Check sheet for the drawn part. Datum: minimum x, y, z corner. Units: mm. A direction names the side the tool comes from. Give positions to 0.01 mm unless a question says otherwise; leave off trailing zeros. Order: outer loops, then holes, each group sorted by start corner. A loop starts at its lowest first (then second) coordinate and runs counter-clockwise, first axis right, second up. Notation, with made-up numbers: M 23,36.5 L 34,36.5 A18 ccw 34,69.5 Z; hole C 21,-9.75 d4. An arc over 180 degrees is marked long. Answer as CSV lines item,"result". Start each with the question number.
Q1. Thickness scan on line 1 (Y direction, x = 6, z = 2.4); line 2 (Y direction, x = 8.25, z = 4.75); line 3 (Z direction, x = 2.75, y = 2). Record the ranges inside material, lowest first.
Q2. Go/stop test with flat-tipped pins: pin 1 (5 mm diameter, centred on y = 4, z = 8.5, fed in from -X); pin 2 (1 mm diameter, centred on x = 4.5, y = 3.5, fed in from +Z); pin 3 (4 mm diameter, centred on x = 2.5, z = 10, fed in from -Y). Record where each tip stops, or that it passes through.
Q3. Mould release check, pull along Z, two halves, no side actions. Record for the marked faces 1, 2 and 3: +Z half, -Z half, draft (parallel to the pull), parting line (faces both ways), or undercut.
Q4. Section check D-D, the plane z = 1.5. Record the boundary of the cut face in (x, y).
Q5. Set-up check for the marked faces 4 and 5: record each of +Z, -Z, +X, -X, +Y, -Y from which the full face is reachable in a straight line by a thin tool's end or side.
Q6. Section check C-C, the plane y = 3.5. Record the boundary of the cut face in (x, z), then the cut area to 3 significant figures.
Q7. Section check B-B, the plane z = 8.75. Record the boundary of the cut face in (x, y).
Q8. Section check A-A, the plane x = 6. Record the boundary of the cut face in (y, z).
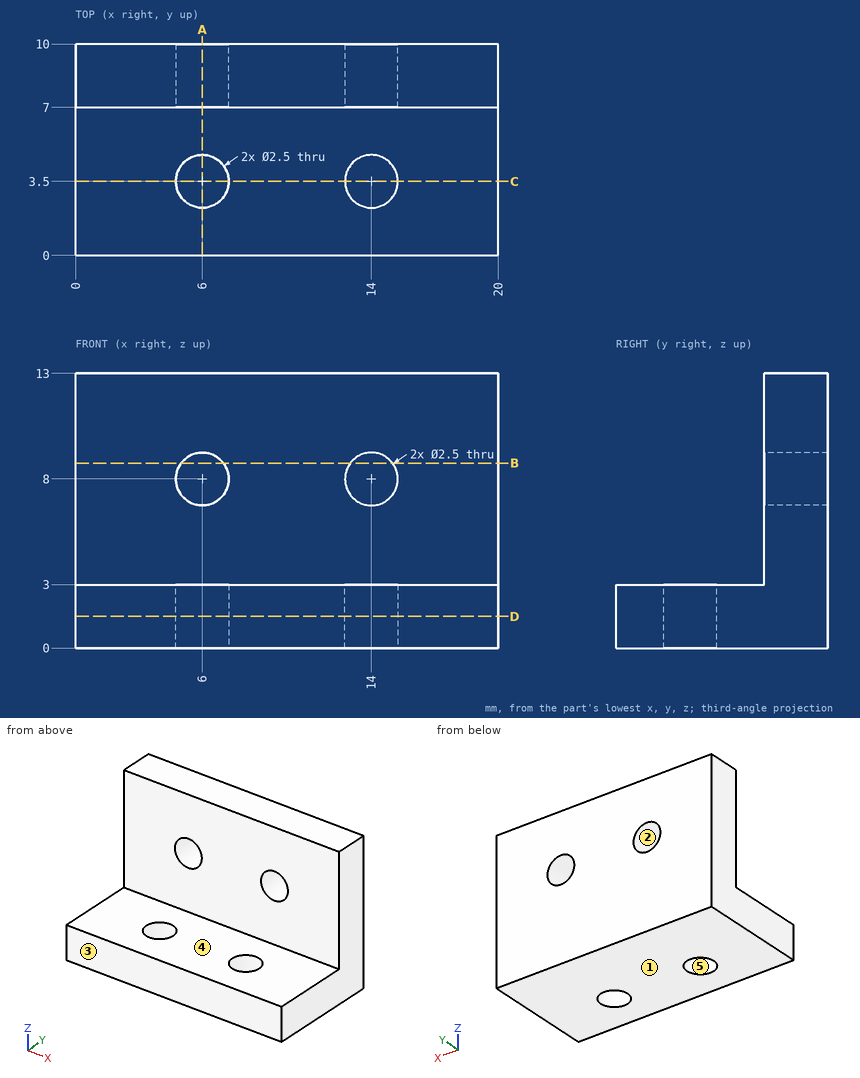
Answer block:
1,line 1,"y = 0 to 2.25, 4.75 to 10"
1,line 2,"y = 7 to 10"
1,line 3,"z = 0 to 3"
2,pin 1,"passes through"
2,pin 2,"stops at z = 3"
2,pin 3,"stops at y = 7"
3,face 1,"-Z half"
3,face 2,"undercut"
3,face 3,"draft"
4,outline,"M 0,0 L 20,0 L 20,10 L 0,10 Z; hole C 6,3.5 d2.5; hole C 14,3.5 d2.5"
5,face 4,"+Z, +X, -X, -Y"
5,face 5,"+Z, -Z"
6,outline,"M 0,0 L 4.75,0 L 4.75,3 L 0,3 Z; M 7.25,0 L 12.75,0 L 12.75,3 L 7.25,3 Z; M 15.25,0 L 20,0 L 20,3 L 15.25,3 Z"
6,area,"45.0 mm2"
7,outline,"M 0,7 L 5,7 L 5,10 L 0,10 Z; M 7,7 L 13,7 L 13,10 L 7,10 Z; M 15,7 L 20,7 L 20,10 L 15,10 Z"
8,outline,"M 0,0 L 2.25,0 L 2.25,3 L 0,3 Z; M 4.75,0 L 10,0 L 10,6.75 L 7,6.75 L 7,3 L 4.75,3 Z; M 7,9.25 L 10,9.25 L 10,13 L 7,13 Z"
